Verification items for the finished model (mm, model axes). Give positions to 0.01 mm unless a question says otherwise; leave off trailing zeros. Loops run counter-clockwise (first coordinate to the right, second up) from the corner with the lowest first, then second, coordinate; pieces in that order, holes last. Notation, with made-up numbers: (8, 53.5) -> (42, 53.5) arc R13 cw to (42, 75.5) -> close; hole circle Ø7 at (46.5, 65). An arc over 180 degrees is marked (long way). Use one line per item in the form item = value. Start each with the question number.
from build123d import *

# Parameters (mm, degrees)
SKETCH2_R           = 1
BOSS_EXTRUDE1_DEPTH = 2
SCALE1_SCALE        = 2


with BuildPart() as part:
    # Sketch2 → Boss-Extrude1 (new body)
    # profile 1 of 4: a face of its own
    with BuildSketch(Plane(origin=(0, 0, 0), x_dir=(1, 0, 0), z_dir=(0, 1, 0))):
        with BuildLine():
            Line((-1.534348462, -5.637537028), (1.534348462, -5.637537028))
            ThreePointArc((1.534348462, -5.637537028), (4.324823338, -6.236497301), (6.623693303, -7.927857797))
            ThreePointArc((6.623693303, -7.927857797), (10.236440266, -7.514468852), (13.78312899, -6.712078584))
            ThreePointArc((13.78312899, -6.712078584), (16.421478173, -5.190969631), (18.558961711, -3.021678736))
            ThreePointArc((18.558961711, -3.021678736), (19.45411943, -1.286546543), (19.346117765, 0.662896123))
            ThreePointArc((19.346117765, 0.662896123), (18.649238809, 4.17439457), (20.639475337, 7.15016677))
            Line((20.639475337, 7.15016677), (17.967387551, 9.159795774))
            ThreePointArc((17.967387551, 9.159795774), (10.858325227, 7.499674132), (4.169484372, 10.424426945))
            Line((4.169484372, 10.424426945), (-4.169484372, 10.424426945))
            ThreePointArc((-4.169484372, 10.424426945), (-10.858325227, 7.499674132), (-17.967387551, 9.159795774))
            Line((-17.967387551, 9.159795774), (-20.639475337, 7.15016677))
            ThreePointArc((-20.639475337, 7.15016677), (-18.649238809, 4.17439457), (-19.346117765, 0.662896123))
            ThreePointArc((-19.346117765, 0.662896123), (-19.45411943, -1.286546543), (-18.558961711, -3.021678736))
            ThreePointArc((-18.558961711, -3.021678736), (-16.421478173, -5.190969631), (-13.78312899, -6.712078584))
            ThreePointArc((-13.78312899, -6.712078584), (-10.236440266, -7.514468852), (-6.623693303, -7.927857797))
            ThreePointArc((-6.623693303, -7.927857797), (-4.324823338, -6.236497301), (-1.534348462, -5.637537028))
        make_face()
        with Locations(Location((-8.5, 0, 0), (0, 0, 270))):
            Circle(SKETCH2_R, mode=Mode.SUBTRACT)
        with Locations(Location((8.5, 0, 0), (0, 0, 270))):
            Circle(SKETCH2_R, mode=Mode.SUBTRACT)
    # profile 2 of 4: a face of its own
    with BuildSketch(Plane(origin=(0, 0, 0), x_dir=(1, 0, 0), z_dir=(0, 1, 0))):
        Polygon((-0.696104526, 13.114793475), (-2.224138848, 10.424426945), (2.224138848, 10.424426945), (0.696104526, 13.114793475), (0, 13.358013588), align=None)
    # profile 3 of 4: a face of its own
    with BuildSketch(Plane(origin=(0, 0, 0), x_dir=(1, 0, 0), z_dir=(0, 1, 0))):
        with BuildLine():
            ThreePointArc((-12.276686285, -7.102440046), (-12.194265553, -8.245293076), (-11.737308023, -9.296052821))
            ThreePointArc((-11.737308023, -9.296052821), (-10.975506649, -9.937799505), (-10.090124565, -10.394175126))
            Line((-10.090124565, -10.394175126), (-7.391598262, -11.698651137))
            Line((-7.391598262, -11.698651137), (-0.775741109, -11.143020661))
            Line((-0.775741109, -11.143020661), (0, -10.959524643))
            Line((0, -10.959524643), (0.775741109, -11.143020661))
            Line((0.775741109, -11.143020661), (7.391598262, -11.698651137))
            Line((7.391598262, -11.698651137), (10.090124565, -10.394175126))
            ThreePointArc((10.090124565, -10.394175126), (10.975506649, -9.937799505), (11.737308023, -9.296052821))
            ThreePointArc((11.737308023, -9.296052821), (12.194265553, -8.245293076), (12.276686285, -7.102440046))
            ThreePointArc((12.276686285, -7.102440046), (9.46781094, -7.635829891), (6.623693303, -7.927857797))
            ThreePointArc((6.623693303, -7.927857797), (4.324823338, -6.236497301), (1.534348462, -5.637537028))
            Line((1.534348462, -5.637537028), (-1.534348462, -5.637537028))
            ThreePointArc((-1.534348462, -5.637537028), (-4.324823338, -6.236497301), (-6.623693303, -7.927857797))
            ThreePointArc((-6.623693303, -7.927857797), (-9.46781094, -7.635829891), (-12.276686285, -7.102440046))
        make_face()
    # profile 4 of 4: a face of its own
    with BuildSketch(Plane(origin=(0, 0, 0), x_dir=(1, 0, 0), z_dir=(0, 1, 0))):
        Polygon((-7.391598262, -11.698651137), (-0.775741109, -11.143020661), (0, -10.959524643), (0.775741109, -11.143020661), (7.391598262, -11.698651137), align=None)
    extrude(amount=BOSS_EXTRUDE1_DEPTH)


with BuildPart() as part_1:
    # Scale1: scaled about (0, 1, 0.244603094)
    add(part.part.scale(SCALE1_SCALE).moved(Location((0, -1, -0.244603094))))


solid = part_1.part
Item 1: Gauge pin test, flat ends, axial feed: pin 1 Ø1 at (x, y) = (-24.5, 2.5) entering from -Z; pin 2 Ø1 at (y, z) = (1.5, -0.5) entering from -X; pin 3 Ø1.9 at (x, y) = (5.5, 1) entering from -Z. Record the tip position at first contact, or that the pin passes through.
Item 2: Sectioned sample at D-D, the plane x = -26. Enter the section's corners in (y, z).
Item 3: Sectioned sample at A-A, the plane z = -16. Enter the section's corners in (x, y).
Item 4: Material ranges on line 1 (Z direction, x = -15.5, y = 2.3); line 2 (X direction, y = 2.3, z = -10.5); line 3 (Z direction, x = -12, y = 2.65), recorded low to high.
Item 5: Draft check along Z on faces 1 (the cylindrical face through (-15.017, 0.972, -0.505)), 2 (the flat face through (-6, 1, -21.093)), 3 (the cylindrical face through (21.928, 0.972, 19.646)). Enter one of: +Z half, -Z half, draft (parallel to the pull), parting line (faces both ways), or undercut.
Item 6: Sectioned sample at C-C, the plane x = 17. Enter the section's corners in (y, z).
Item 7: Sectioned sample at B-B, the plane y = 0.95. Enter the section's corners in (x, z), and give its area (3 significant figures).
Outcome:
q1.pin_1 = -15.18
q1.pin_2 = -39.03
q1.pin_3 = -21.09
q2.outline = (-1, -15.25) -> (3, -15.25) -> (3, 13.6) -> (-1, 13.6) -> close
q3.outline = (-39.34, -1) -> (-30.05, -1) -> (-30.05, 3) -> (-39.34, 3) -> close; (-17.6, -1) -> (17.6, -1) -> (17.6, 3) -> (-17.6, 3) -> close; (30.05, -1) -> (39.34, -1) -> (39.34, 3) -> (30.05, 3) -> close
q4.line_1 = -16.7 to -1.57, 1.08 to 22.81
q4.line_2 = -37.9 to 37.9
q4.line_3 = -18.4 to 23.15
q5.face_1 = undercut
q5.face_2 = -Z half
q5.face_3 = +Z half
q6.outline = (-1, -16.18) -> (3, -16.18) -> (3, -2.24) -> (-1, -2.24) -> close; (-1, 1.76) -> (3, 1.76) -> (3, 22.08) -> (-1, 22.08) -> close
q7.outline = (-41.28, -14.54) -> (-35.93, -18.56) arc R23.15 cw to (-8.34, -21.09) -> (-4.45, -21.09) -> (-1.39, -26.47) -> (0, -26.96) -> (1.39, -26.47) -> (4.45, -21.09) -> (8.34, -21.09) arc R23.15 cw to (35.93, -18.56) -> (41.28, -14.54) arc R9.35 cw to (38.69, -1.57) arc R7.43 ccw to (37.12, 5.8) arc R22.64 ccw to (27.57, 13.18) arc R67.02 ccw to (24.55, 13.96) arc R6.81 ccw to (23.47, 18.35) arc R8.91 ccw to (20.18, 20.54) -> (14.78, 23.15) -> (-14.78, 23.15) -> (-20.18, 20.54) arc R8.91 ccw to (-23.47, 18.35) arc R6.81 ccw to (-24.55, 13.96) arc R67.02 ccw to (-27.57, 13.18) arc R22.64 ccw to (-37.12, 5.8) arc R7.43 ccw to (-38.69, -1.57) arc R9.35 cw to start; hole circle Ø4 at (-17, -0.24); hole circle Ø4 at (17, -0.24)
q7.area = 2,740 mm^2
